from build123d import *

# Parameters (mm, degrees)
SKETCH_3_R      = 1.55
SKETCH_3_W      = 10
SKETCH_3_H      = 3.1
SKETCH_3_W_2    = 3.1
SKETCH_3_H_2    = 10
SKETCH_3_W_3    = 140
SKETCH_3_H_3    = 140
EXTRUDE_1_DEPTH = 3


with BuildPart() as part:
    # 草图3 → 凸台-拉伸1 (new body)
    with BuildSketch(Plane(origin=(0, 0, 0), x_dir=(1, 0, 0), z_dir=(0, 1, 0))):
        with BuildLine():
            ThreePointArc((0, 3), (0.878679656, 0.878679656), (3, 0))
            Line((3, 0), (207, 0))
            ThreePointArc((207, 0), (209.121320344, 0.878679656), (210, 3))
            Line((210, 3), (210, 207))
            ThreePointArc((210, 207), (209.121320344, 209.121320344), (207, 210))
            Line((207, 210), (3, 210))
            ThreePointArc((3, 210), (0.878679656, 209.121320344), (0, 207))
            Line((0, 207), (0, 3))
        make_face()
        with Locations((3, 3)):
            Circle(SKETCH_3_R, mode=Mode.SUBTRACT)
        with Locations((20, 10.35)):
            Rectangle(SKETCH_3_W, SKETCH_3_H, mode=Mode.SUBTRACT)
        with Locations((10.35, 20)):
            Rectangle(SKETCH_3_W_2, SKETCH_3_H_2, mode=Mode.SUBTRACT)
        with Locations((190, 10.35)):
            Rectangle(SKETCH_3_W, SKETCH_3_H, mode=Mode.SUBTRACT)
        with Locations((207, 3)):
            Circle(SKETCH_3_R, mode=Mode.SUBTRACT)
        with Locations((199.65, 20)):
            Rectangle(SKETCH_3_W_2, SKETCH_3_H_2, mode=Mode.SUBTRACT)
        with Locations((105, 196.55)):
            Rectangle(SKETCH_3_W_3, SKETCH_3_H, mode=Mode.SUBTRACT)
        Polygon((11.9, 175), (15, 175), (15, 87), (15, 35), (11.9, 35), align=None, mode=Mode.SUBTRACT)
        with Locations((105, 13.45)):
            Rectangle(SKETCH_3_W_3, SKETCH_3_H, mode=Mode.SUBTRACT)
        with Locations((196.55, 105)):
            Rectangle(SKETCH_3_W_2, SKETCH_3_H_3, mode=Mode.SUBTRACT)
        with Locations((10.35, 190)):
            Rectangle(SKETCH_3_W_2, SKETCH_3_H_2, mode=Mode.SUBTRACT)
        with Locations((3, 207)):
            Circle(SKETCH_3_R, mode=Mode.SUBTRACT)
        with Locations((20, 199.65)):
            Rectangle(SKETCH_3_W, SKETCH_3_H, mode=Mode.SUBTRACT)
        with Locations((199.65, 190)):
            Rectangle(SKETCH_3_W_2, SKETCH_3_H_2, mode=Mode.SUBTRACT)
        with Locations((190, 199.65)):
            Rectangle(SKETCH_3_W, SKETCH_3_H, mode=Mode.SUBTRACT)
        with Locations((207, 207)):
            Circle(SKETCH_3_R, mode=Mode.SUBTRACT)
        with BuildLine():
            ThreePointArc((133, 184.80254627), (134.55, 183.25254627), (133, 181.70254627))
            ThreePointArc((133, 181.70254627), (131.45, 183.25254627), (133, 184.80254627))
        make_face(mode=Mode.SUBTRACT)
        with Locations((155, 183)):
            Circle(SKETCH_3_R, mode=Mode.SUBTRACT)
        with Locations((192, 192)):
            Circle(SKETCH_3_R, mode=Mode.SUBTRACT)
        with Locations((18, 18)):
            Circle(SKETCH_3_R, mode=Mode.SUBTRACT)
        with Locations((55, 27)):
            Circle(SKETCH_3_R, mode=Mode.SUBTRACT)
        with Locations((77, 27)):
            Circle(SKETCH_3_R, mode=Mode.SUBTRACT)
        with Locations((27, 55)):
            Circle(SKETCH_3_R, mode=Mode.SUBTRACT)
        with Locations((27, 77)):
            Circle(SKETCH_3_R, mode=Mode.SUBTRACT)
        with Locations((133, 27)):
            Circle(SKETCH_3_R, mode=Mode.SUBTRACT)
        with Locations((155, 27)):
            Circle(SKETCH_3_R, mode=Mode.SUBTRACT)
        with Locations((192, 18)):
            Circle(SKETCH_3_R, mode=Mode.SUBTRACT)
        with Locations((183, 55)):
            Circle(SKETCH_3_R, mode=Mode.SUBTRACT)
        with Locations((183, 77)):
            Circle(SKETCH_3_R, mode=Mode.SUBTRACT)
        with Locations((27, 133)):
            Circle(SKETCH_3_R, mode=Mode.SUBTRACT)
        with Locations((27, 155)):
            Circle(SKETCH_3_R, mode=Mode.SUBTRACT)
        with Locations((18, 192)):
            Circle(SKETCH_3_R, mode=Mode.SUBTRACT)
        with Locations((55, 183)):
            Circle(SKETCH_3_R, mode=Mode.SUBTRACT)
        with Locations((77, 183)):
            Circle(SKETCH_3_R, mode=Mode.SUBTRACT)
        with Locations((183, 133)):
            Circle(SKETCH_3_R, mode=Mode.SUBTRACT)
        with Locations((183, 155)):
            Circle(SKETCH_3_R, mode=Mode.SUBTRACT)
    extrude(amount=EXTRUDE_1_DEPTH)


solid = part.part
The model under review builds one solid part; all positions refer to its coordinate system, in mm. Round coordinates to 2 decimals unless told otherwise and drop trailing zeros. Loops run counter-clockwise (first coordinate to the right, second up) from the corner with the lowest first, then second, coordinate; pieces in that order, holes last. Notation, with made-up numbers: (54, -23.75) -> (86, -23.75) arc R23 ccw to (86, 7.25) -> close; hole circle Ø11 at (69.5, -14). An arc over 180 degrees is marked (long way). Return JSON: item names as keys, results as strings.
(1) For line 1 (X direction, y = 1.6, z = -183); line 2 (Z direction, x = 188, y = 1.2); line 3 (Z direction, x = 79, y = 0.65), list the stretches that pass through material, from the lowest coordinate up.
Solved:
{"line 1": "0 to 53.45, 56.55 to 75.45, 78.55 to 131.47, 134.53 to 153.45, 156.55 to 210", "line 2": "-210 to -201.2, -198.1 to -11.9, -8.8 to 0", "line 3": "-210 to -198.1, -195 to -15, -11.9 to 0"}
(2) Add section A-A on x = 104. Write out the cut boundary in (y, z), plus the area to 3 significant figures.
Solved:
{"outline": "(0, -210) -> (3, -210) -> (3, -198.1) -> (0, -198.1) -> close; (0, -195) -> (3, -195) -> (3, -15) -> (0, -15) -> close; (0, -11.9) -> (3, -11.9) -> (3, 0) -> (0, 0) -> close", "area": "611 mm2"}
(3) Add section C-C on y = 2.25. State how many separate pieces and enclosed holes the cut face has, plus the area to 3 significant figures.
Solved:
{"separate pieces": "1", "enclosed holes": "36", "area": "41,900 mm2"}
(4) For pin 1 (4 mm diameter, centred on x = 3, z = -207, fed in from -Y), flat-tipped, find the tip position at first contact; note if it passes through.
Solved:
{"pin 1": "y = 0"}
(5) Add section B-B on z = -123. Write out the cut boundary in (x, y).
Solved:
{"outline": "(0, 0) -> (11.9, 0) -> (11.9, 3) -> (0, 3) -> close; (15, 0) -> (195, 0) -> (195, 3) -> (15, 3) -> close; (198.1, 0) -> (210, 0) -> (210, 3) -> (198.1, 3) -> close"}
